CAD build for the part. Positions are in the model's coordinates, mm. Give positions to 0.01 mm unless a question says otherwise; leave off trailing zeros. Order: outer loops, then holes, each group sorted by start corner. A loop starts at its lowest first (then second) coordinate and runs counter-clockwise, first axis right, second up. Notation, with made-up numbers: (39, 73.25) -> (90, 73.25) arc R15 ccw to (90, 92.25) -> close; hole circle Ø5 at (64.25, 41.25). An arc over 180 degrees is marked (long way). Answer as CSV lines item,"result".
```python
from build123d import *

# Parameters (mm, degrees)
SKETCH_1_R         = 45
EXTRUDE_1_DEPTH    = 0.5
FILLET_3_R         = 0.2
DOME_2_FACE_RADIUS = 44.8
DOME_2_HEIGHT      = 10


with BuildPart() as part:
    # Эскиз1 → Бобышка-Вытянуть1 (new body)
    with BuildSketch(Plane(origin=(0, 0, 0), x_dir=(1, 0, 0), z_dir=(0, 1, 0))):
        with Locations(Location((0, 0, 0), (0, 0, 270))):
            Circle(SKETCH_1_R)
    extrude(amount=EXTRUDE_1_DEPTH)

    # Скругление3
    fillet_3_edges = [part.edges().sort_by_distance(p)[0] for p in [
        (0, 0, -45),
    ]]
    fillet(fillet_3_edges, radius=FILLET_3_R)

    # Купол2: a dome of height H over a round flat face of radius A is a cap of a sphere of radius (A * A + H * H) / (2 * H)
    dome_2_r = (DOME_2_FACE_RADIUS * DOME_2_FACE_RADIUS + DOME_2_HEIGHT * DOME_2_HEIGHT) / (2 * DOME_2_HEIGHT)
    dome_2_base = Plane((0, 0, 0), z_dir=(0, -1, 0))
    with Locations(dome_2_base.offset(DOME_2_HEIGHT - dome_2_r)):
        dome_2_ball = Sphere(dome_2_r, mode=Mode.PRIVATE)
    add(split(dome_2_ball, bisect_by=dome_2_base, keep=Keep.TOP, mode=Mode.PRIVATE))


solid = part.part
```
1) Pin check, flat tips, straight feed: P1, Ø8, axis at x = -28, z = 21, coming from the -Y side; P2, Ø8, axis at x = 13.5, z = -9, coming from the -Y side; P3, Ø3, axis at y = -1, z = -7, coming from the -X side. Stop position of each tip, or through.
Data:
P1,"stops at y = -5.34"
P2,"stops at y = -9.29"
P3,"stops at x = -44.59"
2) Wall check: line 1 along Y through (x, z) = (-16, 39); line 2 along Y through (x, z) = (9, -26); line 3 along X through (y, z) = (0.25, -37). Give the ranges that are in metal, low to high. Write a range as [from, to].
Data:
line 1,"y = [-1.2, 0.5]"
line 2,"y = [-6.34, 0.5]"
line 3,"x = [-25.61, 25.61]"
3) Band-saw the part on C-C, the plane y = -2.25. Write the cut outline in (x, z), then the cut area to 3 significant figures.
Data:
outline,"circle Ø79.32 at (0, 0)"
area,"4,940 mm2"
4) Band-saw the part on B-B, the plane x = 0. Write the cut outline in (y, z).
Data:
outline,"(0, -44.8) arc R0.2 ccw to (0.2, -45) -> (0.5, -45) -> (0.5, 45) -> (0.2, 45) arc R0.2 ccw to (0, 44.8) arc R105.35 ccw to start"
5) Band-saw the part on A-A, the plane z = 0. Write the cut outline in (x, y).
Data:
outline,"(-45, 0.2) arc R0.2 ccw to (-44.8, 0) arc R105.35 ccw to (44.8, 0) arc R0.2 ccw to (45, 0.2) -> (45, 0.5) -> (-45, 0.5) -> close"
